Could you check a few things on this drawing? It's one solid part, dimensions in mm from its lowest x, y, z. Coordinates: 2 decimals unless noted, no trailing zeros. Order: outer loops, then holes, each group sorted by start corner. A loop starts at its lowest first (then second) coordinate and runs counter-clockwise, first axis right, second up. Notation, with made-up numbers: (57, 53.5) - (66, 53.5) arc R16 ccw to (66, 79.5) - close; hole circle Ø2 at (68, 79). An arc over 180 degrees is marked (long way). Answer in a Markdown table with one row per item. Add a question column.
Item 1: Will these pins go through, and if not, where does the flat tip stop? pin 1 Ø0.8 at (x, y) = (11, 0.5) entering from +Z; pin 2 Ø1.4 at (x, y) = (44.5, 0.5) entering from +Z (3 decimals); pin 3 Ø1.5 at (x, y) = (26.5, 2) entering from -Z (3 decimals).
Item 2: If I drill on line 1 along Z through (x, y) = (23, 0.7) (3 decimals); line 2 along X through (y, z) = (1.75, 29.5) (3 decimals); line 3 along X through (y, z) = (0.1, 208.5), over which ranges is the centre line in solid material (lowest first)? Write a range as from..to.
Item 3: I want a section at A-A (y = 0.85). Please give me the cut outline in (x, z) (3 decimals), plus the area to 3 significant figures.
Item 4: I want a section at C-C (x = 33). Please give me the cut outline in (y, z) (3 decimals), plus the area to 3 significant figures.
Item 5: I want a section at B-B (z = 35.5). Please give me the cut outline in (x, y) (3 decimals).
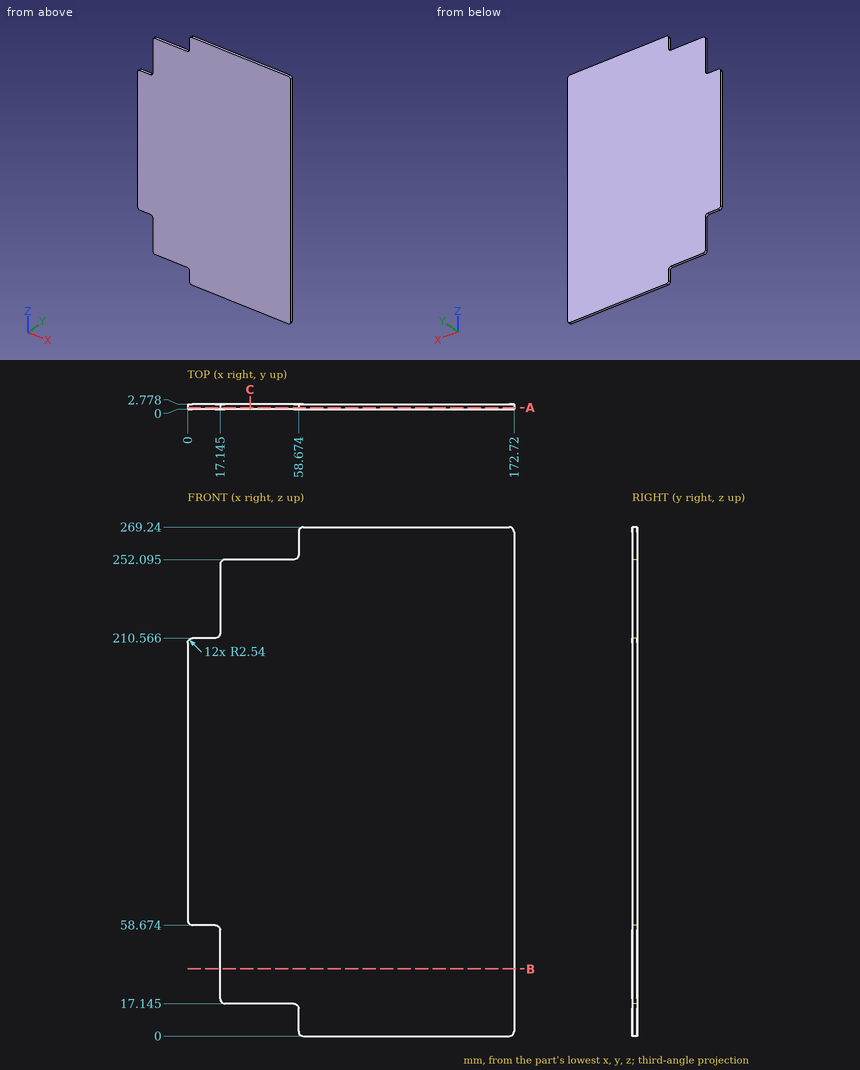
Values follow:
| question | item | result |
|---|---|---|
| 1 | pin 1 | stops at z = 210.57 |
| 1 | pin 2 | stops at z = 252.095 |
| 1 | pin 3 | stops at z = 17.145 |
| 2 | line 1 | z = 17.145..252.095 |
| 2 | line 2 | x = 17.145..172.72 |
| 2 | line 3 | x = 0.04..172.72 |
| 3 | outline | (0, 61.214) arc R2.54 ccw to (2.54, 58.674) - (14.605, 58.674) arc R2.54 cw to (17.145, 56.134) - (17.145, 19.685) arc R2.54 ccw to (19.685, 17.145) - (56.134, 17.145) arc R2.54 cw to (58.674, 14.605) - (58.674, 2.54) arc R2.54 ccw to (61.214, 0) - (170.18, 0) arc R2.54 ccw to (172.72, 2.54) - (172.72, 266.7) arc R2.54 ccw to (170.18, 269.24) - (61.214, 269.24) arc R2.54 ccw to (58.674, 266.7) - (58.674, 254.635) arc R2.54 cw to (56.134, 252.095) - (19.685, 252.095) arc R2.54 ccw to (17.145, 249.555) - (17.145, 213.106) arc R2.54 cw to (14.605, 210.566) - (2.54, 210.566) arc R2.54 ccw to (0, 208.026) - close |
| 3 | area | 43,100 mm^2 |
| 4 | outline | (0, 17.145) - (2.778, 17.145) - (2.778, 252.095) - (0, 252.095) - close |
| 4 | area | 653 mm^2 |
| 5 | outline | (17.145, 0) - (172.72, 0) - (172.72, 2.778) - (17.145, 2.778) - close |
